Geometry: final body of the model. Coordinates: model frame, mm. Face numbers are marked on the shaded views. A direction names the side the tool comes from. Coordinates: 2 decimals unless noted, no trailing zeros. Loops run counter-clockwise (first coordinate to the right, second up) from the corner with the lowest first, then second, coordinate; pieces in that order, holes last. Notation, with made-up numbers: (80.5, -31.75) - (90.5, -31.75) arc R16 cw to (90.5, -9.75) - close; hole circle Ø8 at (76.5, 86). An arc over 180 degrees is marked (long way). Answer in a Markdown table with one row per item.
from build123d import *

# Parameters (mm, degrees)
SKETCH1_W           = 38.1
SKETCH1_H           = 76.2
BOSS_EXTRUDE1_DEPTH = 7.9375
SKETCH2_R           = 3.96875
CUT_EXTRUDE1_DEPTH  = 44.330317403
SKETCH4_R           = 9.525
CUT_EXTRUDE2_DEPTH  = 4.7625
SKETCH5_R           = 5.08
BOSS_EXTRUDE2_DEPTH = 9.4488
SKETCH6_R           = 3.302
CUT_EXTRUDE3_DEPTH  = 47.008650575
SKETCH7_W           = 38.1
SKETCH7_H           = 31.75
SKETCH7_R           = 2
BOSS_EXTRUDE4_DEPTH = 7.9375


with BuildPart() as part:
    # Sketch1 → Boss-Extrude1 (new body)
    with BuildSketch(Plane.XY):
        Rectangle(SKETCH1_W, SKETCH1_H)
    extrude(amount=BOSS_EXTRUDE1_DEPTH)

    # Sketch2 → Cut-Extrude1 (cut, through all)
    with BuildSketch(Plane.XY.offset(7.9375)):
        Circle(SKETCH2_R)
    extrude(amount=-CUT_EXTRUDE1_DEPTH, mode=Mode.SUBTRACT)

    # Sketch4 → Cut-Extrude2 (cut)
    with BuildSketch(Plane.XY.offset(7.9375)):
        Circle(SKETCH4_R)
    extrude(amount=-CUT_EXTRUDE2_DEPTH, mode=Mode.SUBTRACT)

    # Sketch5 → Boss-Extrude2 (add)
    with BuildSketch(Plane.XY.offset(7.9375)):
        with Locations(Location((0, 25.4, 0), (0, 0, 180))):
            Circle(SKETCH5_R)
    boss_extrude2 = extrude(amount=BOSS_EXTRUDE2_DEPTH)

    # Sketch6 → Cut-Extrude3 (cut, through all)
    with BuildSketch(Plane.XY.offset(17.3863)):
        with Locations((0, 25.4)):
            Circle(SKETCH6_R)
    cut_extrude3 = extrude(amount=-CUT_EXTRUDE3_DEPTH, mode=Mode.SUBTRACT)

    # Mirror1: Boss-Extrude2, Cut-Extrude3 across plane
    add(boss_extrude2.mirror(Plane.ZX))
    add(cut_extrude3.mirror(Plane.ZX), mode=Mode.SUBTRACT)

    # Sketch7 → Boss-Extrude4 (add)
    with BuildSketch(Plane.XY.offset(7.9375)):
        with Locations((0, 53.975)):
            Rectangle(SKETCH7_W, SKETCH7_H)
        with Locations((-12.7, 63.5)):
            Circle(SKETCH7_R, mode=Mode.SUBTRACT)
        with Locations(Location((-12.7, 44.45, 0), (0, 0, 180))):
            Circle(SKETCH7_R, mode=Mode.SUBTRACT)
    extrude(amount=-BOSS_EXTRUDE4_DEPTH)


solid = part.part
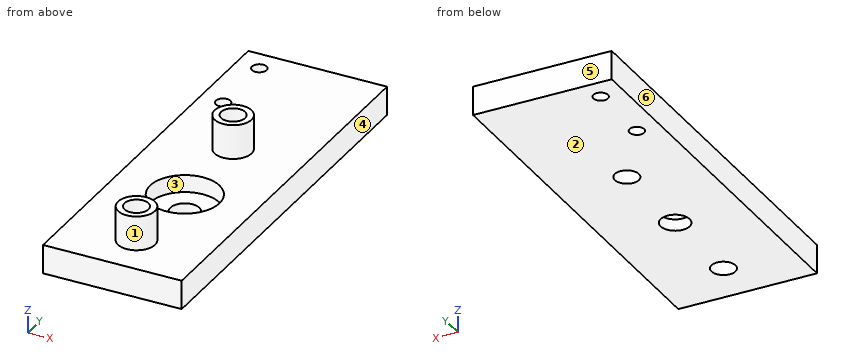
(1) Access query for the marked faces 1 and 2. Directions: +Z, -Z, +X, -X, +Y, -Y. A direction counts if a zero-diameter tool reaches every point of the face in a straight line with its end or side. Return the directions, or none.
Verdict:
| item | result |
|---|---|
| face 1 | +Z |
| face 2 | -Z, +X, -X, +Y, -Y |
(2) Cut plane B-B on x = -12.7. Output: boundary loops of the cut face in (y, z), then the cut area to 3 significant figures.
Verdict:
| item | result |
|---|---|
| outline | (-38.1, 0) - (42.45, 0) - (42.45, 7.94) - (-38.1, 7.94) - close; (46.45, 0) - (61.5, 0) - (61.5, 7.94) - (46.45, 7.94) - close; (65.5, 0) - (69.85, 0) - (69.85, 7.94) - (65.5, 7.94) - close |
| area | 793 mm² |
(3) Cut plane C-C on z = 11.75. Output: boundary loops of the cut face in (x, y).
Verdict:
| item | result |
|---|---|
| outline | circle Ø10.16 at (0, -25.4); circle Ø10.16 at (0, 25.4); hole circle Ø6.6 at (0, -25.4); hole circle Ø6.6 at (0, 25.4) |
(4) First-contact query: pin 1 Ø7.5 at (x, y) = (0, 25.4) entering from +Z; pin 2 Ø3 at (x, y) = (5.5, 8.5) entering from +Z; pin 3 Ø12.5 at (x, y) = (0, 0) entering from +Z (3 decimals). Flat tips, straight axial feed; report the tip coordinate or a pass-through.
Verdict:
| item | result |
|---|---|
| pin 1 | stops at z = 17.39 |
| pin 2 | stops at z = 7.94 |
| pin 3 | stops at z = 3.175 |
(5) Pull-direction query (X, two-part tool) for the marked faces 3, 4, 5 and 6; classes: pulls with the +X half, pulls with the -X half, needs draft (parallel to the pull), parting line crosses it, or undercut.
Verdict:
| item | result |
|---|---|
| face 3 | undercut |
| face 4 | pulls with the +X half |
| face 5 | needs draft |
| face 6 | pulls with the -X half |
(6) Ray query, probe 1 along Y at (x, z) = (-12.7, 5.75); probe 2 along Y at (x, z) = (0, 6.1) (3 decimals); probe 3 along Y at (x, z) = (0, 10.75). Return the intervals inside material, ascending.
Verdict:
| item | result |
|---|---|
| probe 1 | y = -38.1 to 42.45, 46.45 to 61.5, 65.5 to 69.85 |
| probe 2 | y = -38.1 to -28.702, -22.098 to -9.525, 9.525 to 22.098, 28.702 to 69.85 |
| probe 3 | y = -30.48 to -28.7, -22.1 to -20.32, 20.32 to 22.1, 28.7 to 30.48 |
(7) Cut plane D-D on x = 0. State how many separate pieces and enclosed holes the cut face has, then the cut area to 3 significant figures.
Verdict:
| item | result |
|---|---|
| separate pieces | 4 |
| enclosed holes | 0 |
| area | 703 mm² |
